Here's how the part is built. I have some questions about the finished solid (model axes, mm). A direction names the side the tool comes from. Give positions to 0.01 mm unless a question says otherwise; leave off trailing zeros. Loops run counter-clockwise (first coordinate to the right, second up) from the corner with the lowest first, then second, coordinate; pieces in that order, holes last. Notation, with made-up numbers: (68, 35.25) - (101, 35.25) arc R22 cw to (101, 64.25) - close; hole circle Ø5 at (44, -27). An arc over 180 degrees is marked (long way). Return JSON: item names as keys, results as strings. Group by question number.
(1) For P1, Ø1.5, axis at x = -62.5, z = 13.5, coming from the -Y side; P2, Ø4.5, axis at y = 139, z = -11.5, coming from the -X side; P3, Ø14, axis at x = 0, y = 218, coming from the +Z side; P4, Ø12, axis at x = 22, z = -35, coming from the -Y side, each with a flat end and sliding along its axis, tell me the tip position at first contact or that it passes through.
(2) If we section it at A-A (z = 0): State how many separate pieces and enclosed holes the cut face has, then the cut area to 3 significant figures.
(3) If we section it at B-B (y = 138.5): Please give me the cut outline in (x, z).
(4) On a 3-axis mill with a long thin cutter (end or side, diameter ignored), from which of +Z, -Z, +X, -X, +Y, -Y can I reach the whole of each face in a straight line? I mean faces 5 (the flat face through (82, 6, 49)), 6 (the cylindrical face through (-58, 127, 0)), 7 (the flat face through (-48, 102, -10)), 8 (the flat face through (-30, 127, 18)), 9 (the flat face through (52, 114, 10)). Say none if no direction works.
(5) I need wall thicknesses on probe 1 along X at (y, z) = (9.25, -45); probe 2 along X at (y, z) = (168, -11.75); probe 3 along X at (y, z) = (2, -45). Which ranges of each line are inside material? Lowest first, please. Write a range as [from, to].
(6) If we mould it in two halves opening along Y, with no side actions, what happens to faces 1 (the flat face through (1, 5, 0)), 2 (the flat face through (-30, 127, -18)), 3 (the cylindrical face through (58, 127, 0)), 4 (the cylindrical face through (-50.202, 175.436, 14.056))? For each: released by +Y, released by -Y, zero draft, split by the parting line, or undercut.
(7) If we section it at C-C (y = 218): Please give me the cut outline in (x, z).
(8) If we section it at D-D (z = 42): Please give me the cut outline in (x, y).
```python
from build123d import *

# Parameters (mm, degrees)
BOSS_EXTRUDE1_DEPTH                      = 19
CBORE_FOR_M6_HEX_HEAD_BOLT1_D            = 15
CBORE_FOR_M6_HEX_HEAD_BOLT1_CBORE_D      = 20
CBORE_FOR_M6_HEX_HEAD_BOLT1_CBORE_DEPTH  = 13
BOSS_EXTRUDE2_DEPTH                      = 36
CUT_EXTRUDE1_DEPTH                       = 36
CBORE_FOR_M16_HEX_HEAD_BOLT1_D           = 17.5
CBORE_FOR_M16_HEX_HEAD_BOLT1_DEPTH       = 41
CBORE_FOR_M16_HEX_HEAD_BOLT1_CBORE_D     = 22
CBORE_FOR_M16_HEX_HEAD_BOLT1_CBORE_DEPTH = 15
CBORE_FOR_M5_HEX_HEAD_BOLT1_D            = 12
CBORE_FOR_M5_HEX_HEAD_BOLT1_CBORE_D      = 15
CBORE_FOR_M5_HEX_HEAD_BOLT1_CBORE_DEPTH  = 8
SKETCH9_W                                = 60
SKETCH9_H                                = 5
CUT_EXTRUDE2_DEPTH                       = 301.481280615
F_10_0MM_DOWEL_HOLE1_D                   = 10
F_10_0MM_DOWEL_HOLE1_DEPTH               = 36
F_10_0MM_DOWEL_HOLE1_TIP                 = 3.004303095
CUT_EXTRUDE3_START                       = -8
SKETCH12_R                               = 7.5
CUT_EXTRUDE3_DEPTH                       = 8


with BuildPart() as part:
    # Sketch1 → Boss-Extrude1 (new body)
    with BuildSketch(Plane(origin=(0, 0, 0), x_dir=(1, 0, 0), z_dir=(0, 1, 0))):
        with BuildLine():
            Line((-75, -60), (75, -60))
            ThreePointArc((75, -60), (85.606601718, -55.606601718), (90, -45))
            Line((90, -45), (90, 45))
            ThreePointArc((90, 45), (85.606601718, 55.606601718), (75, 60))
            Line((75, 60), (-75, 60))
            ThreePointArc((-75, 60), (-85.606601718, 55.606601718), (-90, 45))
            Line((-90, 45), (-90, -45))
            ThreePointArc((-90, -45), (-85.606601718, -55.606601718), (-75, -60))
        make_face()
    extrude(amount=BOSS_EXTRUDE1_DEPTH)

    # CBORE for M6 Hex Head Bolt1 (through all)
    with Locations(Plane(origin=(-75, 19, 45), x_dir=(0, 0, 1), z_dir=(0, 1, 0))):
        with Locations((0, 0), (-90, 0), (-90, 150), (0, 150)):
            CounterBoreHole(CBORE_FOR_M6_HEX_HEAD_BOLT1_D / 2, CBORE_FOR_M6_HEX_HEAD_BOLT1_CBORE_D / 2, CBORE_FOR_M6_HEX_HEAD_BOLT1_CBORE_DEPTH)

    # Sketch3 → Boss-Extrude2 (add)
    with BuildSketch(Plane.XY.offset(18)):
        with BuildLine():
            Line((-65, 168), (-65, 0))
            Line((-65, 0), (65, 0))
            Line((65, 0), (65, 168))
            ThreePointArc((65, 168), (0, 233), (-65, 168))
        make_face()
    extrude(amount=-BOSS_EXTRUDE2_DEPTH)

    # Sketch4 → Cut-Extrude1 (cut)
    with BuildSketch(Plane.XY.offset(18)):
        with BuildLine():
            Line((24, 142.524521594), (24, 133.475478406))
            ThreePointArc((24, 133.475478406), (0, 73), (-24, 133.475478406))
            Line((-24, 133.475478406), (-24, 142.524521594))
            ThreePointArc((-24, 142.524521594), (0, 203), (24, 142.524521594))
        make_face()
    extrude(amount=-CUT_EXTRUDE1_DEPTH, mode=Mode.SUBTRACT)

    # CBORE for M16 Hex Head Bolt1
    with Locations(Plane(origin=(65, 138, 0), x_dir=(0, 1, 0), z_dir=(1, 0, 0))):
        with Locations((0, 0)):
            cbore_for_m16_hex_head_bolt1 = CounterBoreHole(CBORE_FOR_M16_HEX_HEAD_BOLT1_D / 2, CBORE_FOR_M16_HEX_HEAD_BOLT1_CBORE_D / 2, CBORE_FOR_M16_HEX_HEAD_BOLT1_CBORE_DEPTH, depth=CBORE_FOR_M16_HEX_HEAD_BOLT1_DEPTH)

    # Mirror1: CBORE for M16 Hex Head Bolt1 across plane
    add(cbore_for_m16_hex_head_bolt1.mirror(Plane(origin=(0, 0, 0), x_dir=(0, 0, 1), z_dir=(1, 0, 0))), mode=Mode.SUBTRACT)

    # CBORE for M5 Hex Head Bolt1 (through all)
    with Locations(Plane(origin=(0, 218, 18), x_dir=(1, 0, 0), z_dir=(0, 0, 1))):
        with Locations((0, 0), (-49.225256247, -50), (-49.687709551, -110), (0, -160), (49.897824361, -110), (49.991173273, -50)):
            CounterBoreHole(CBORE_FOR_M5_HEX_HEAD_BOLT1_D / 2, CBORE_FOR_M5_HEX_HEAD_BOLT1_CBORE_D / 2, CBORE_FOR_M5_HEX_HEAD_BOLT1_CBORE_DEPTH)

    # Sketch9 → Cut-Extrude2 (cut, through all)
    with BuildSketch(Plane(origin=(90, 0, 0), x_dir=(0, 0, -1), z_dir=(1, 0, 0))):
        with Locations((0, 2.5)):
            Rectangle(SKETCH9_W, SKETCH9_H)
    extrude(amount=-CUT_EXTRUDE2_DEPTH, mode=Mode.SUBTRACT)

    # Ø10.0mm Dowel Hole1
    with Locations(Plane(origin=(35.355339059, 203.355339059, 18), x_dir=(1, 0, 0), z_dir=(0, 0, 1))):
        with Locations((0, 0), (-70.710678118, -130.710678118)):
            Hole(F_10_0MM_DOWEL_HOLE1_D / 2, depth=F_10_0MM_DOWEL_HOLE1_DEPTH)
            with Locations((0, 0, -(F_10_0MM_DOWEL_HOLE1_DEPTH + F_10_0MM_DOWEL_HOLE1_TIP / 2))):  # 118° drill point
                Cone(0, F_10_0MM_DOWEL_HOLE1_D / 2, F_10_0MM_DOWEL_HOLE1_TIP, mode=Mode.SUBTRACT)

    # Sketch12 → Cut-Extrude3 (cut)
    with BuildSketch(Plane(origin=(0, 0, -18), x_dir=(-1, 0, 0), z_dir=(0, 0, -1)).offset(CUT_EXTRUDE3_START)):
        with Locations(Location((0, 218, 0), (0, 0, 180))):
            Circle(SKETCH12_R)
        with Locations(Location((-49.991173273, 168, 0), (0, 0, 180))):
            Circle(SKETCH12_R)
        with Locations(Location((-49.897824361, 108, 0), (0, 0, 180))):
            Circle(SKETCH12_R)
        with Locations(Location((49.687709551, 108, 0), (0, 0, 180))):
            Circle(SKETCH12_R)
        with Locations(Location((49.225256247, 168, 0), (0, 0, 180))):
            Circle(SKETCH12_R)
        with Locations(Location((0, 58, 0), (0, 0, 180))):
            Circle(SKETCH12_R)
    extrude(amount=CUT_EXTRUDE3_DEPTH, mode=Mode.SUBTRACT)


solid = part.part
```
Values:
{
 "1": {"P1": "y = 5", "P2": "x = -65", "P3": "z = 10", "P4": "y = 0"},
 "2": {"separate pieces": "2", "enclosed holes": "8", "area": "18,700 mm2"},
 "3": {"outline": "(-65, -18) - (-24, -18) - (-24, -8.74) - (-50, -8.74) - (-50, -10.99) - (-65, -10.99) - close; (-65, 10.99) - (-50, 10.99) - (-50, 8.74) - (-24, 8.74) - (-24, 18) - (-65, 18) - close; (24, -18) - (65, -18) - (65, -10.99) - (50, -10.99) - (50, -8.74) - (24, -8.74) - close; (24, 8.74) - (50, 8.74) - (50, 10.99) - (65, 10.99) - (65, 18) - (24, 18) - close"},
 "4": {"face 5": "+Y", "face 6": "-X", "face 7": "-Z", "face 8": "+Z, +X, -X, +Y", "face 9": "+Z"},
 "5": {"probe 1": "[-90, -85], [-65, 65], [85, 90]", "probe 2": "[-65, -56.73], [-41.73, -35], [35, 42.49], [57.49, 65]", "probe 3": "[-90, -82.5], [-67.5, 67.5], [82.5, 90]"},
 "6": {"face 1": "released by -Y", "face 2": "zero draft", "face 3": "undercut", "face 4": "undercut"},
 "7": {"outline": "(-41.53, -18) - (-7.5, -18) - (-7.5, -10) - (-6, -10) - (-6, 10) - (-7.5, 10) - (-7.5, 18) - (-41.53, 18) - close; (6, -10) - (7.5, -10) - (7.5, -18) - (41.53, -18) - (41.53, 18) - (7.5, 18) - (7.5, 10) - (6, 10) - close"},
 "8": {"outline": "(-90, 0) - (-81.87, 0) - (-81.87, 6) - (-84.54, 6) - (-84.54, 19) - (-90, 19) - close; (-68.13, 0) - (68.13, 0) - (68.13, 6) - (65.46, 6) - (65.46, 19) - (-65.46, 19) - (-65.46, 6) - (-68.13, 6) - close; (81.87, 0) - (90, 0) - (90, 19) - (84.54, 19) - (84.54, 6) - (81.87, 6) - close"}
}
